Check sheet for the modelled part. Datum: model origin and axes. Units: mm. Give positions to 0.01 mm unless a question says otherwise; leave off trailing zeros. Write each loop counter-clockwise with the first axis right and the second up, starting at its lowest first coordinate (ties: lowest second). Pieces come first, ordered by that corner, then holes. Notation, with made-up numbers: M 19,9 L 75,9 A20 cw 75,48 Z; hole C 62,-36.5 d1. An arc over 180 degrees is marked long. Write item = value, one per line. Start each with the question number.
1) Sectioned sample at B-B, the plane x = 15.25. Record the cut outline in (y, z).
2) Gauge pin test, flat ends, axial feed: pin 1 (3 mm diameter, centred on x = 8, y = 1, fed in from -Z); pin 2 (0.8 mm diameter, centred on x = 4.5, z = 1, fed in from -Y). Record the tip position at first contact, or that the pin passes through.
3) Sectioned sample at D-D, the plane y = -1. Record the cut outline in (x, z).
4) Sectioned sample at C-C, the plane z = 0.35. Count the separate pieces of the cut face and the enclosed holes in it, then the cut area to 3 significant figures.
5) Scan lines: L1, parallel to Y at x = 3.5, z = 1; L2, parallel to Y at x = -0.75, z = 0.95; L3, parallel to Y at x = 15.5, z = 0.85. Record each from-to range of solid material in increasing order.
6) Sectioned sample at A-A, the plane x = 3.5. Record the cut outline in (y, z), then the cut area to 3 significant figures.
from build123d import *

# Parameters (mm, degrees)
SKETCH_R  = 0.8
PAD_DEPTH = 1.5


with BuildPart() as part:
    # Sketch → Pad (new body)
    with BuildSketch(Plane.XY):
        with BuildLine():
            Line((12.124356, 21), (2.124356, 21))
            add(Edge.make_bspline(
                [(-2.5, 33.5), (2.301311, 30.873257), (2.124356, 21)],
                knots=[0, 0, 0, 1, 1, 1], degree=2))
            add(Edge.make_bspline(
                [(2.572068, 36), (-0.563366, 35.88435), (-2.5, 33.5)],
                knots=[0, 0, 0, 1, 1, 1], degree=2))
            Line((2.572068, 36), (12.572068, 36))
            Line((12.572068, 36), (23.212256, 29.991259))
            Line((23.212256, 29.991259), (17.554762, 21.745486))
            Line((17.554762, 21.745486), (-0.84276, -10.119957))
            Line((-0.84276, -10.119957), (-5.84276, -10.119957))
            Line((-5.84276, -10.119957), (12.124356, 21))
        make_face()
        with Locations((9, 22.5)):
            Circle(SKETCH_R, mode=Mode.SUBTRACT)
        with Locations((9, 34.5)):
            Circle(SKETCH_R, mode=Mode.SUBTRACT)
        with Locations((15.5, 29)):
            Circle(SKETCH_R, mode=Mode.SUBTRACT)
        with Locations((-1.039206, -6.119957)):
            Circle(SKETCH_R, mode=Mode.SUBTRACT)
        with Locations((7.960794, 9.4685)):
            Circle(SKETCH_R, mode=Mode.SUBTRACT)
        with Locations((3.460794, 1.674271)):
            Circle(SKETCH_R, mode=Mode.SUBTRACT)
    extrude(amount=PAD_DEPTH)


solid = part.part
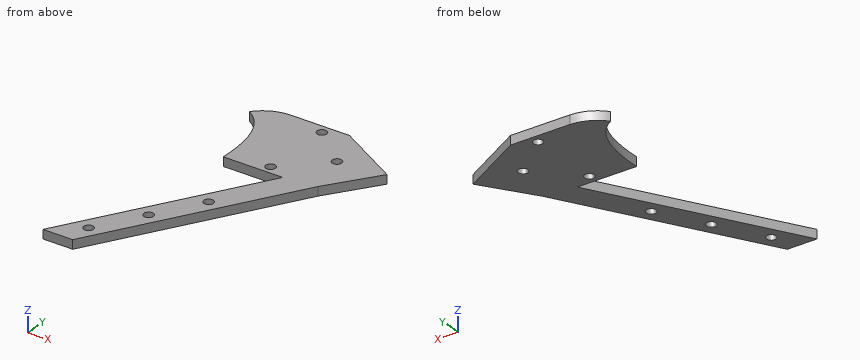
Data:
q1.outline = M 17.75,0 L 28.24,0 L 28.24,1.5 L 17.75,1.5 Z; M 29.76,0 L 34.49,0 L 34.49,1.5 L 29.76,1.5 Z
q2.pin_1 = through
q2.pin_2 = -1.56
q3.outline = M -0.58,0 L 4.42,0 L 4.42,1.5 L -0.58,1.5 Z
q4.separate_pieces = 1
q4.enclosed_holes = 6
q4.area = 421 mm2
q5.L1 = -2.6 to 0.88, 2.47 to 6.06, 21 to 36
q5.L2 = -9.96 to -6.87, -5.37 to -1.3, 32.13 to 35.05
q5.L3 = 18.19 to 28.2, 29.8 to 34.35
q6.outline = M -2.6,0 L 0.88,0 L 0.88,1.5 L -2.6,1.5 Z; M 2.47,0 L 6.06,0 L 6.06,1.5 L 2.47,1.5 Z; M 21,0 L 36,0 L 36,1.5 L 21,1.5 Z
q6.area = 33.1 mm2
